Here's how the part is built. I have some questions about the finished solid (model axes, mm). A direction names the side the tool comes from. Coordinates: 2 decimals unless noted, no trailing zeros. Write each loop counter-clockwise with the first axis right and the second up, starting at its lowest first coordinate (ties: lowest second). Pieces come first, ordered by that corner, then holes.
Item 1: If we section it at D-D (x = 39): Please give me the cut outline in (y, z).
Item 2: For faces 1 (the face through (42, -19, 4)), 2 (the face through (-41, 27.5, 3)), 3 (the face through (-40, -8, 3)), which set-ups out of +Z, -Z, +X, -X, +Y, -Y let a thin tool reach every point of the face, with its end or its side?
Item 3: I'm going to push flat-ended pins straight in: pin 1 Ø3 at (x, y) = (27, 21.5) entering from +Z; pin 2 Ø2 at (y, z) = (21.5, 7.5) entering from +X; pin 3 Ø0.8 at (y, z) = (17, 0.5) entering from -X. Where does each tip first touch, or does it pass through?
Item 4: We'd pull the mould along Y, two halves only. Please class faces 4 (the face through (37, -24, 9.5)), 5 (the face through (1, 29, 3)): +Y half, -Y half, draft (parallel to the pull), parting line (faces both ways), or undercut.
Item 5: If I drill on line 1 (Y direction, x = 39, z = 4); line 2 (X direction, y = 24.5, z = 4.25); line 3 (Y direction, x = 39, z = 6.75), over which ranges is the centre line in solid material (lowest first)?
Item 6: If we section it at B-B (x = 6): Please give me the cut outline in (y, z), then the cut area to 3 significant figures.
Item 7: If we section it at A-A (x = -11): Please give me the cut outline in (y, z).
Item 8: If we section it at C-C (y = -2): Please give me the cut outline in (x, z), then the cut area to 3 significant figures.
from build123d import *

# Parameters (mm, degrees)
SKETCH_W        = 3
SKETCH_H        = 21
PAD_DEPTH       = 1
SKETCH001_W     = 5
SKETCH001_H     = 1.75
SKETCH001_H_2   = 1
PAD001_DEPTH    = 5
SKETCH002_W     = 3
SKETCH002_H     = 1
PAD002_DEPTH    = 2
SKETCH003_R     = 2.5
SKETCH003_R_2   = 1.3
PAD003_DEPTH    = 8.5
SKETCH004_W     = 16
SKETCH004_H     = 3.5
POCKET_DEPTH    = 1
CHAMFER_SIZE    = 0.5
SKETCH005_W     = 3
SKETCH005_H     = 1
PAD004_DEPTH    = 7
SKETCH006_W     = 56
SKETCH006_H     = 7
POCKET001_DEPTH = 9.501


with BuildPart() as part:
    # Sketch → Pad (new body)
    with BuildSketch(Plane.XY):
        Polygon((-45, 30), (45, 30), (45, -30), (-45, -30), (-45, -26.25), (-22, -26.25), (-22, -9.25), (-45, -9.25), (-45, -7.5), (-27, -7.5), (-27, 9.5), (-45, 9.5), (-45, 10.5), (-27, 10.5), (-27, 27.5), (-45, 27.5), align=None)
        Polygon((36.5, 21), (36.5, 28), (-16.5, 28), (-16.5, 21), (7, 21), (7, 19), (13, 19), (13, 21), align=None, mode=Mode.SUBTRACT)
        with Locations((5.5, 0)):
            Rectangle(SKETCH_W, SKETCH_H, mode=Mode.SUBTRACT)
        with Locations((11.5, 0)):
            Rectangle(SKETCH_W, SKETCH_H, mode=Mode.SUBTRACT)
        with Locations((17.5, 0)):
            Rectangle(SKETCH_W, SKETCH_H, mode=Mode.SUBTRACT)
        with Locations((23.5, 0)):
            Rectangle(SKETCH_W, SKETCH_H, mode=Mode.SUBTRACT)
    extrude(amount=PAD_DEPTH)

    # Sketch001 (on Face42 of Pad) → Pad001 (join)
    with BuildSketch(Plane.XY.offset(1)):
        with Locations((-42.5, -8.375)):
            Rectangle(SKETCH001_W, SKETCH001_H)
        with Locations((-42.5, 10)):
            Rectangle(SKETCH001_W, SKETCH001_H_2)
        Polygon((-45, 30), (45, 30), (45, -30), (-45, -30), (-45, -26.25), (-40, -26.25), (-40, -29), (40, -29), (40, -27.5), (43.5, -27.5), (43.5, 27.5), (40, 27.5), (40, 29), (-40, 29), (-40, 27.5), (-45, 27.5), align=None)
    extrude(amount=PAD001_DEPTH)

    # Sketch002 (on Face56 of Pad001) → Pad002 (join)
    with BuildSketch(Plane.XY.offset(6)):
        with Locations((41.5, 28)):
            Rectangle(SKETCH002_W, SKETCH002_H)
        with Locations((-41.5, 28)):
            Rectangle(SKETCH002_W, SKETCH002_H)
        with Locations((-41.5, -28)):
            Rectangle(SKETCH002_W, SKETCH002_H)
        with Locations((41.5, -28)):
            Rectangle(SKETCH002_W, SKETCH002_H)
    extrude(amount=PAD002_DEPTH)

    # Sketch003 (on Face47 of Pad002) → Pad003 (join)
    with BuildSketch(Plane.XY.offset(1)):
        with Locations((-19, 24.5)):
            Circle(SKETCH003_R)
        with Locations((-19, 24.5)):
            Circle(SKETCH003_R_2, mode=Mode.SUBTRACT)
        with Locations((39, 24.5)):
            Circle(SKETCH003_R)
        with Locations((39, 24.5)):
            Circle(SKETCH003_R_2, mode=Mode.SUBTRACT)
        with Locations((-19, -24.5)):
            Circle(SKETCH003_R)
        with Locations((-19, -24.5)):
            Circle(SKETCH003_R_2, mode=Mode.SUBTRACT)
        with Locations((39, -24.5)):
            Circle(SKETCH003_R)
        with Locations((39, -24.5)):
            Circle(SKETCH003_R_2, mode=Mode.SUBTRACT)
    extrude(amount=PAD003_DEPTH)

    # Sketch004 (on Face45 of Pad003) → Pocket (cut)
    with BuildSketch(Plane.XZ.offset(30)):
        with BuildLine():
            ThreePointArc((-14.5, 6), (-11, 2.5), (-7.5, 6))
            Line((-14.5, 6), (-7.5, 6))
        make_face()
        with Locations((10.5, 4.25)):
            Rectangle(SKETCH004_W, SKETCH004_H)
    extrude(amount=-POCKET_DEPTH, mode=Mode.SUBTRACT)

    # Chamfer
    chamfer_edges = [part.edges().sort_by_distance(p)[0] for p in [
        (-20.3, 24.5, 9.5),
        (37.7, 24.5, 9.5),
        (-20.3, -24.5, 9.5),
        (37.7, -24.5, 9.5),
    ]]
    chamfer(chamfer_edges, length=CHAMFER_SIZE)

    # Sketch005 (on Face5 of Chamfer) → Pad004 (join)
    with BuildSketch(Plane.XY.offset(1)):
        with Locations((42, -16.2)):
            Rectangle(SKETCH005_W, SKETCH005_H)
        with Locations((42, -19.5)):
            Rectangle(SKETCH005_W, SKETCH005_H)
    extrude(amount=PAD004_DEPTH)

    # Sketch006 (on Face63 of Pad004) → Pocket001 (cut, through all)
    with BuildSketch(Plane(origin=(0, 0, 0), x_dir=(1, 0, 0), z_dir=(0, 0, -1))):
        with Locations((10, -24.5)):
            Rectangle(SKETCH006_W, SKETCH006_H)
    extrude(amount=-POCKET001_DEPTH, mode=Mode.SUBTRACT)


solid = part.part
Answer list:
1. outline: (-30, 0) - (30, 0) - (30, 6) - (29, 6) - (29, 1) - (27, 1) - (27, 9.5) - (26.3, 9.5) - (25.8, 9) - (25.8, 1) - (23.2, 1) - (23.2, 9) - (22.7, 9.5) - (22, 9.5) - (22, 1) - (-22, 1) - (-22, 9.5) - (-22.7, 9.5) - (-23.2, 9) - (-23.2, 1) - (-25.8, 1) - (-25.8, 9) - (-26.3, 9.5) - (-27, 9.5) - (-27, 1) - (-29, 1) - (-29, 6) - (-30, 6) - close
2. face 1: +Z, -X
2. face 2: +Z, -Z, -X
2. face 3: +Z
3. pin 1: stops at z = 1
3. pin 2: stops at x = 40.5
3. pin 3: stops at x = -27
4. face 4: draft
4. face 5: undercut
5. line 1: y = -30 to -29, -27 to -25.8, -23.2 to -22, 22 to 23.2, 25.8 to 27, 29 to 30
5. line 2: x = -21.5 to -20.3, 40.3 to 41.5, 43.5 to 45
5. line 3: y = -27 to -25.8, -23.2 to -22, 22 to 23.2, 25.8 to 27
6. outline: (-30, 0) - (-10.5, 0) - (-10.5, 1) - (-29, 1) - (-29, 2.5) - (-30, 2.5) - close; (10.5, 0) - (21, 0) - (21, 1) - (10.5, 1) - close; (28, 0) - (30, 0) - (30, 6) - (29, 6) - (29, 1) - (28, 1) - close
6. area: 38.5 mm2
7. outline: (-30, 0) - (21, 0) - (21, 1) - (-29, 1) - (-29, 2.5) - (-30, 2.5) - close; (28, 0) - (30, 0) - (30, 6) - (29, 6) - (29, 1) - (28, 1) - close
8. outline: (-27, 0) - (4, 0) - (4, 1) - (-27, 1) - close; (7, 0) - (10, 0) - (10, 1) - (7, 1) - close; (13, 0) - (16, 0) - (16, 1) - (13, 1) - close; (19, 0) - (22, 0) - (22, 1) - (19, 1) - close; (25, 0) - (45, 0) - (45, 6) - (43.5, 6) - (43.5, 1) - (25, 1) - close
8. area: 67.5 mm2
